```python
from build123d import *

# Parameters (mm, degrees)
SKETCH_1_R          = 2.5
EXTRUDE_1_DEPTH     = 3
SKETCH_3_R          = 1
CUT_EXTRUDE_1_DEPTH = 20.02771451


with BuildPart() as part:
    # 草圖1 → 填料-伸長1 (new body)
    with BuildSketch(Plane(origin=(0, 0, 0), x_dir=(1, 0, 0), z_dir=(0, 1, 0))):
        with BuildLine():
            Line((-16.25468329, 1.404493766), (0, 7.5))
            Line((0, 7.5), (16.25468329, 1.404493766))
            ThreePointArc((16.25468329, 1.404493766), (17.227998127, 0), (16.25468329, -1.404493766))
            Line((16.25468329, -1.404493766), (0, -7.5))
            Line((0, -7.5), (-16.25468329, -1.404493766))
            ThreePointArc((-16.25468329, -1.404493766), (-17.227998127, 0), (-16.25468329, 1.404493766))
        make_face()
        with Locations(Location((0, 0, 0), (0, 0, 270))):
            Circle(SKETCH_1_R, mode=Mode.SUBTRACT)
    extrude(amount=EXTRUDE_1_DEPTH)

    # 草圖3 → 除料-伸長1 (cut, through all)
    with BuildSketch(Plane(origin=(0, 3, 0), x_dir=(1, 0, 0), z_dir=(0, 1, 0))):
        with Locations(Location((15.727998127, 0, 0), (0, 0, 270))):
            Circle(SKETCH_3_R)
    extrude(amount=-CUT_EXTRUDE_1_DEPTH, mode=Mode.SUBTRACT)


solid = part.part
```
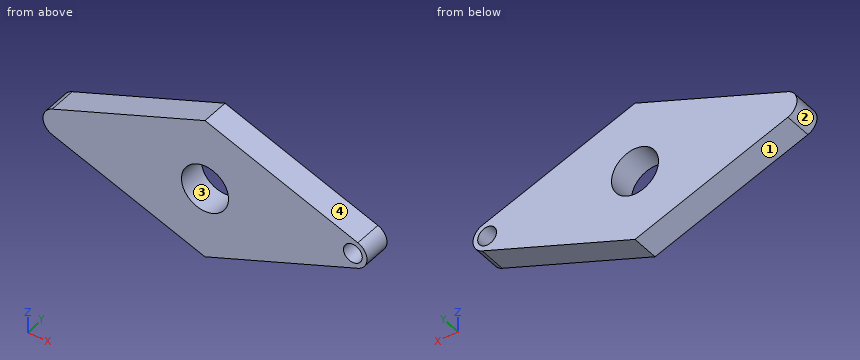
CAD build for the part. Positions are in the model's coordinates, mm. Face numbers are marked on the shaded views. Give positions to 0.01 mm unless a question says otherwise; leave off trailing zeros. Order: outer loops, then holes, each group sorted by start corner. A loop starts at its lowest first (then second) coordinate and runs counter-clockwise, first axis right, second up.
(1) Flat gauge pin, fed straight in: pin 1 (1 mm diameter, centred on y = 2.5, z = -1.5, fed in from +X). Where does the tip first touch, or does it go through?
(2) Mould opens along Z. For the marked faces 1, 2, 3 and 4 say: released by +Z, released by -Z, zero draft, split by the parting line, or undercut.
(3) Drill centre lines: L1, parallel to X at y = 1, z = 0; L2, parallel to X at y = 0.7, z = -0.5; L3, parallel to Z at x = 1, y = 2 (3 decimals). Where is each one in solid material? Low to high.
(4) Saw through at B-B, the plane x = 0.5. Give the cut face in (y, z), then the cut area to 3 significant figures.
(5) Saw through at D-D, the plane x = -8. Give the cut face in (y, z), then the cut area to 3 significant figures.
(6) Saw through at C-C, the plane y = 0.85. Give the cut face in (x, z).
(7) Saw through at A-A, the plane z = 0. Give the cut face in (x, y), then the cut area to 3 significant figures.
Results found:
1. pin 1: stops at x = 16.85
2. face 1: released by -Z
2. face 2: split by the parting line
2. face 3: undercut
2. face 4: released by +Z
3. L1: x = -17.23 to -2.5, 2.5 to 14.73, 16.73 to 17.23
3. L2: x = -17.14 to -2.45, 2.45 to 14.86, 16.59 to 17.14
3. L3: z = -7.125 to -2.291, 2.291 to 7.125
4. outline: (0, -7.31) - (3, -7.31) - (3, -2.45) - (0, -2.45) - close; (0, 2.45) - (3, 2.45) - (3, 7.31) - (0, 7.31) - close
4. area: 29.2 mm2
5. outline: (0, -4.5) - (3, -4.5) - (3, 4.5) - (0, 4.5) - close
5. area: 27.0 mm2
6. outline: (-16.25, -1.4) - (0, -7.5) - (16.25, -1.4) arc R1.5 ccw to (16.25, 1.4) - (0, 7.5) - (-16.25, 1.4) arc R1.5 ccw to start; hole circle Ø5 at (0, 0); hole circle Ø2 at (15.73, 0)
7. outline: (-17.23, 0) - (-2.5, 0) - (-2.5, 3) - (-17.23, 3) - close; (2.5, 0) - (14.73, 0) - (14.73, 3) - (2.5, 3) - close; (16.73, 0) - (17.23, 0) - (17.23, 3) - (16.73, 3) - close
7. area: 82.4 mm2
